```python
from build123d import *

# Parameters (mm, degrees)
EXTRUDE_1_DEPTH          = 37.5
SHELL_START              = -33.5
SHELL_1_DEPTH            = 67
FILLET_1_R               = 5
FILLET_3_R               = 2
FILLET_4_R               = 1
CUT_EXTRUDE_2_DEPTH      = 94.307288033
CUT_EXTRUDE_2_DEPTH_BACK = 3
SKETCH_3_R               = 1.9
CUT_EXTRUDE_1_DEPTH      = 103.419810201
CUT_EXTRUDE_1_DEPTH_BACK = 103.419810201
SKETCH_2_W               = 80
SKETCH_2_H               = 27
CUT_EXTRUDE_3_REACH      = 102.177
SKETCH_4_R               = 1.8


# Read off the part's stored shape, not the designer's step: 抽壳1
with BuildPart() as part:
    # 草图1 → 凸台-拉伸1 (new, symmetric)
    with BuildSketch(Plane(origin=(0, 0, 0), x_dir=(0, 0, -1), z_dir=(1, 0, 0))):
        Polygon((-70.540010176, 52.231309316), (-70.540010176, 30), (-80, 30), (-80, 0), (0, 0), (0, 30), (-9.459989824, 30), align=None)
    extrude(amount=EXTRUDE_1_DEPTH, both=True)

    # 抽壳1 outline → 抽壳1 (cut)
    with BuildSketch(Plane.YZ.offset(SHELL_START)):
        Polygon((47.974598226, 70.540010176), (22, 70.540010176), (22, 80), (4, 80), (4, 6), (24.483955603, 6), align=None)
    extrude(amount=SHELL_1_DEPTH, mode=Mode.SUBTRACT)

    # 圆角1
    fillet_1_edges = [part.edges().sort_by_distance(p)[0] for p in [
        (0, 30, 9.459989824),
        (35.5, 30, 70.540010176),
        (-35.5, 30, 70.540010176),
    ]]
    fillet(fillet_1_edges, radius=FILLET_1_R)

    # 圆角3
    fillet_3_edges = [part.edges().sort_by_distance(p)[0] for p in [
        (33.5, 4, 43),
        (33.5, 36.229276914, 38.270005088),
        (-33.5, 36.229276914, 38.270005088),
        (-33.5, 4, 43),
    ]]
    fillet(fillet_3_edges, radius=FILLET_3_R)

    # 圆角4
    fillet_4_edges = [part.edges().sort_by_distance(p)[0] for p in [
        (-37.5, 30, 4.28917746),
        (-37.5, 30.075961235, 9.446595809),
        (37.5, 30, 4.28917746),
        (37.5, 30.075961235, 9.446595809),
        (-37.5, 41.266423106, 40.414232907),
        (0, 52.231309316, 70.540010176),
        (37.5, 41.266423106, 40.414232907),
        (37.5, 0, 40),
        (-37.5, 0, 40),
        (0, 0, 80),
        (0, 0, 0),
        (0, 30, 0),
        (0, 30, 80),
    ]]
    fillet(fillet_4_edges, radius=FILLET_4_R)

    # 草图3 → 切除-拉伸2 (cut, two sides: drawn at the far end of the back side and taken through both)
    with BuildSketch(Plane(origin=(0, 30, 0), x_dir=(1, 0, 0), z_dir=(0, 1, 0)).offset(-CUT_EXTRUDE_2_DEPTH_BACK)):
        with Locations(Location((-32, -4.78917746, 0), (0, 0, 90))):
            Circle(SKETCH_3_R)
        with Locations(Location((32, -4.78917746, 0), (0, 0, 90))):
            Circle(SKETCH_3_R)
        with Locations(Location((0, -75.540010176, 0), (0, 0, 90))):
            Circle(SKETCH_3_R)
    extrude(amount=CUT_EXTRUDE_2_DEPTH + CUT_EXTRUDE_2_DEPTH_BACK, mode=Mode.SUBTRACT)

    # 草图2 → 切除-拉伸1 (cut, two sides: drawn at the far end of the back side and taken through both)
    with BuildSketch(Plane(origin=(0, 0, 0), x_dir=(0, 0, -1), z_dir=(1, 0, 0)).offset(-CUT_EXTRUDE_1_DEPTH_BACK)):
        with Locations((-40, 13.5)):
            Rectangle(SKETCH_2_W, SKETCH_2_H)
    extrude(amount=CUT_EXTRUDE_1_DEPTH + CUT_EXTRUDE_1_DEPTH_BACK, mode=Mode.SUBTRACT)

    # 草图4 → 切除-拉伸3 (cut, up to next)
    with BuildSketch(Plane(origin=(0, 19.69151404, -7.167124978), x_dir=(1, 0, 0), z_dir=(0, -0.9396926207859104, 0.34202014332566316)), mode=Mode.PRIVATE) as cut_extrude_3_sk1:
        with Locations(Location((-18, 75.900768948, 0), (0, 0, 270))):
            Circle(SKETCH_4_R)
    cut_extrude_3_tool1 = extrude(cut_extrude_3_sk1.sketch, amount=-CUT_EXTRUDE_3_REACH, mode=Mode.PRIVATE) & part.part
    # 草图4 → 切除-拉伸3 (cut, up to next)
    with BuildSketch(Plane(origin=(0, 19.69151404, -7.167124978), x_dir=(1, 0, 0), z_dir=(0, -0.9396926207859104, 0.34202014332566316)), mode=Mode.PRIVATE) as cut_extrude_3_sk2:
        with Locations(Location((18, 75.900768948, 0), (0, 0, 270))):
            Circle(SKETCH_4_R)
    cut_extrude_3_tool2 = extrude(cut_extrude_3_sk2.sketch, amount=-CUT_EXTRUDE_3_REACH, mode=Mode.PRIVATE) & part.part
    # 草图4 → 切除-拉伸3 (cut, up to next)
    with BuildSketch(Plane(origin=(0, 19.69151404, -7.167124978), x_dir=(1, 0, 0), z_dir=(0, -0.9396926207859104, 0.34202014332566316)), mode=Mode.PRIVATE) as cut_extrude_3_sk3:
        with Locations(Location((-18, 27.900768948, 0), (0, 0, 270))):
            Circle(SKETCH_4_R)
    cut_extrude_3_tool3 = extrude(cut_extrude_3_sk3.sketch, amount=-CUT_EXTRUDE_3_REACH, mode=Mode.PRIVATE) & part.part
    # 草图4 → 切除-拉伸3 (cut, up to next)
    with BuildSketch(Plane(origin=(0, 19.69151404, -7.167124978), x_dir=(1, 0, 0), z_dir=(0, -0.9396926207859104, 0.34202014332566316)), mode=Mode.PRIVATE) as cut_extrude_3_sk4:
        with Locations(Location((18, 27.900768948, 0), (0, 0, 270))):
            Circle(SKETCH_4_R)
    cut_extrude_3_tool4 = extrude(cut_extrude_3_sk4.sketch, amount=-CUT_EXTRUDE_3_REACH, mode=Mode.PRIVATE) & part.part
    add(cut_extrude_3_tool1.solids().sort_by_distance((-18, 45.651106, 64.156268))[0], mode=Mode.SUBTRACT)
    add(cut_extrude_3_tool2.solids().sort_by_distance((18, 45.651106, 64.156268))[0], mode=Mode.SUBTRACT)
    add(cut_extrude_3_tool3.solids().sort_by_distance((-18, 29.234139, 19.051022))[0], mode=Mode.SUBTRACT)
    add(cut_extrude_3_tool4.solids().sort_by_distance((18, 29.234139, 19.051022))[0], mode=Mode.SUBTRACT)


solid = part.part
```
The listing builds one solid part. Answer for the finished solid, in the listing's coordinates (mm). A direction names the side the tool comes from. Round coordinates to 2 decimals unless told otherwise and drop trailing zeros. Loops run counter-clockwise (first coordinate to the right, second up) from the corner with the lowest first, then second, coordinate; pieces in that order, holes last.
1) Given P1, Ø4, axis at x = 3.5, z = 4, coming from the +Y side; P2, Ø1.5, axis at x = -10, y = 30, coming from the +Z side; P3, Ø4, axis at x = -16, z = 26.5, coming from the -Y side, each flat-ended and moving along its own axis, determine where each tip first touches the part or whether it passes through.
Outcome:
P1: stops at y = 30
P2: stops at z = 79.97
P3: stops at y = 31.22
2) A cutting plane is placed at B-B on x = 0. Determine the outline of the cut face in (y, z), plus the area to 3 significant figures.
Outcome:
outline: (27, 0) - (29, 0) arc R1 ccw to (30, 1) - (30, 8.58) arc R5 cw to (30.3, 10.29) - (51.74, 69.2) arc R1 ccw to (50.8, 70.54) - (47.97, 70.54) - (27, 12.91) - close; (27, 70.54) - (30, 70.54) - (30, 73.64) - (27, 73.64) - close; (27, 77.44) - (30, 77.44) - (30, 79) arc R1 ccw to (29, 80) - (27, 80) - close
area: 302 mm2
3) Consider line 1 (X direction, y = 32.25, z = 70); line 2 (Y direction, x = -8.5, z = 10); line 3 (Y direction, x = 14, z = 27.5). Determine where each line is inside the solid, lowest interval first.
Outcome:
line 1: x = -37.5 to -33.5, 33.5 to 37.5
line 2: y = 27 to 30.21
line 3: y = 32.31 to 36.57
4) A cutting plane is placed at A-A on x = 28.5. Determine the outline of the cut face in (y, z), plus the area to 3 significant figures.
Outcome:
outline: (27, 0) - (29, 0) arc R1 ccw to (30, 1) - (30, 8.58) arc R5 cw to (30.3, 10.29) - (51.74, 69.2) arc R1 ccw to (50.8, 70.54) - (47.97, 70.54) - (27, 12.91) - close; (27, 70.54) - (30, 70.54) - (30, 79) arc R1 ccw to (29, 80) - (27, 80) - close
area: 314 mm2
5) For faces 4 (the face through (1, 30, 73)), 5 (the face through (1, 30, 5)), 6 (the face through (0, 29, 70.54)), determine the directions among +Z, -Z, +X, -X, +Y, -Y from which every point of the face is accessible in a straight line to the end or side of a thin tool.
Outcome:
face 4: +Z, +Y
face 5: -Z, +X, -X, +Y
face 6: -Y
6) For a pull along X with two mould halves and no side action, classify faces 1 (the face through (35.53, 31.5, 71.97)), 2 (the face through (37.215, 41.063, 40.735)), 3 (the face through (19.785, 31.167, 18.597)) as released by +X, released by -X, zero draft, split by the parting line, or undercut.
Outcome:
face 1: zero draft
face 2: released by +X
face 3: undercut
